from build123d import *

# Parameters (mm, degrees)
SKETCH1_R           = 3.2512
SKETCH1_R_2         = 1.27
BOSS_EXTRUDE1_DEPTH = 0.800000051


with BuildPart() as part:
    # Sketch1 → Boss-Extrude1 (new body)
    with BuildSketch(Plane.XY):
        with BuildLine():
            ThreePointArc((21.253467287, -26.289), (46.841342124, -13.11656107), (18.612068966, -7.516505446))
            ThreePointArc((18.612068966, -7.516505446), (15.875, -9.08244408), (13.137931034, -7.516505446))
            ThreePointArc((13.137931034, -7.516505446), (-15.091342124, -13.11656107), (10.496532713, -26.289))
            Line((10.496532713, -26.289), (21.253467287, -26.289))
        make_face()
        with Locations(Location((31.75, -15.24, 0), (0, 0, 180))):
            Circle(SKETCH1_R, mode=Mode.SUBTRACT)
        with Locations(Location((0, -15.24, 0), (0, 0, 180))):
            Circle(SKETCH1_R, mode=Mode.SUBTRACT)
        with Locations(Location((-11.733270063, -10.379920409, 0), (0, 0, 180))):
            Circle(SKETCH1_R_2, mode=Mode.SUBTRACT)
        with Locations(Location((11.733270063, -10.379920409, 0), (0, 0, 180))):
            Circle(SKETCH1_R_2, mode=Mode.SUBTRACT)
        with Locations(Location((-4.860079591, -3.506729937, 0), (0, 0, 180))):
            Circle(SKETCH1_R_2, mode=Mode.SUBTRACT)
        with Locations(Location((4.860079591, -3.506729937, 0), (0, 0, 180))):
            Circle(SKETCH1_R_2, mode=Mode.SUBTRACT)
        with Locations(Location((20.016729937, -10.379920409, 0), (0, 0, 180))):
            Circle(SKETCH1_R_2, mode=Mode.SUBTRACT)
        with Locations(Location((43.483270063, -10.379920409, 0), (0, 0, 180))):
            Circle(SKETCH1_R_2, mode=Mode.SUBTRACT)
        with Locations(Location((26.889920409, -3.506729937, 0), (0, 0, 180))):
            Circle(SKETCH1_R_2, mode=Mode.SUBTRACT)
        with Locations(Location((36.610079591, -3.506729937, 0), (0, 0, 180))):
            Circle(SKETCH1_R_2, mode=Mode.SUBTRACT)
        with Locations(Location((36.610079591, -26.973270063, 0), (0, 0, 180))):
            Circle(SKETCH1_R_2, mode=Mode.SUBTRACT)
        with Locations(Location((20.016729937, -20.100079591, 0), (0, 0, 180))):
            Circle(SKETCH1_R_2, mode=Mode.SUBTRACT)
        with Locations(Location((43.483270063, -20.100079591, 0), (0, 0, 180))):
            Circle(SKETCH1_R_2, mode=Mode.SUBTRACT)
        with Locations(Location((-4.860079591, -26.973270063, 0), (0, 0, 180))):
            Circle(SKETCH1_R_2, mode=Mode.SUBTRACT)
        with Locations(Location((4.860079591, -26.973270063, 0), (0, 0, 180))):
            Circle(SKETCH1_R_2, mode=Mode.SUBTRACT)
        with Locations(Location((-11.733270063, -20.100079591, 0), (0, 0, 180))):
            Circle(SKETCH1_R_2, mode=Mode.SUBTRACT)
        with Locations(Location((11.733270063, -20.100079591, 0), (0, 0, 180))):
            Circle(SKETCH1_R_2, mode=Mode.SUBTRACT)
        with Locations(Location((26.889920409, -26.973270063, 0), (0, 0, 180))):
            Circle(SKETCH1_R_2, mode=Mode.SUBTRACT)
    extrude(amount=BOSS_EXTRUDE1_DEPTH)


solid = part.part
Model file for the job. Use its own axes, mm. Give positions to 0.01 mm unless a question says otherwise; leave off trailing zeros. Order: outer loops, then holes, each group sorted by start corner. A loop starts at its lowest first (then second) coordinate and runs counter-clockwise, first axis right, second up. Notation, with made-up numbers: (60.25, 52.5) - (113.25, 52.5) arc R9 cw to (113.25, 59.5) - close; hole circle Ø3 at (64, 72). An arc over 180 degrees is marked (long way). Return JSON: item names as keys, results as strings.
1) Probe line 1 (Y direction, x = 37, z = 0.65); line 2 (X direction, y = -15.24, z = 0.45); line 3 (X direction, y = -4, z = 0.75). List the from-to ranges inside material, lowest first. Write a range as from..to.
Geometry says:
{"line 1": "-29.55..-28.18, -25.76..-4.72, -2.3..-0.93", "line 2": "-15.24..-3.25, 3.25..28.5, 35..46.99", "line 3": "-10.29..-6.03, -3.69..3.69, 6.03..10.29, 21.46..25.72, 28.06..35.44, 37.78..42.04"}
2) Cut at A-A, the plane y = -15.24. Give the cut face in (x, z).
Geometry says:
{"outline": "(-15.24, 0) - (-3.25, 0) - (-3.25, 0.8) - (-15.24, 0.8) - close; (3.25, 0) - (28.5, 0) - (28.5, 0.8) - (3.25, 0.8) - close; (35, 0) - (46.99, 0) - (46.99, 0.8) - (35, 0.8) - close"}
3) Pull direction Y, two halves, no side cores. Call faces 1 (the cylindrical face through (2.396, -17.437, 0.394)), 2 (the cylindrical face through (15.921, -9.082, 0.394)), 3 (the cylindrical face through (46.9, -13.6, 0.4)): pulls with the +Y half, pulls with the -Y half, needs draft (parallel to the pull), parting line crosses it, or undercut.
Geometry says:
{"face 1": "undercut", "face 2": "pulls with the +Y half", "face 3": "parting line crosses it"}
4) Cut at D-D, the plane y = -19.5. Give the cut face in (x, z), plus the area to 3 significant figures.
Geometry says:
{"outline": "(-14.63, 0) - (-12.85, 0) - (-12.85, 0.8) - (-14.63, 0.8) - close; (-10.61, 0) - (10.61, 0) - (10.61, 0.8) - (-10.61, 0.8) - close; (12.85, 0) - (18.9, 0) - (18.9, 0.8) - (12.85, 0.8) - close; (21.14, 0) - (42.36, 0) - (42.36, 0.8) - (21.14, 0.8) - close; (44.6, 0) - (46.38, 0) - (46.38, 0.8) - (44.6, 0.8) - close", "area": "41.6 mm²"}
5) Cut at C-C, the plane z = 0.5. Count the separate pieces of the cut face and the enclosed holes in it, plus the area to 3 significant figures.
Geometry says:
{"separate pieces": "1", "enclosed holes": "18", "area": "1,370 mm²"}
6) Cut at B-B, the plane x = 31.75. Give the cut face in (y, z), plus the area to 3 significant figures.
Geometry says:
{"outline": "(-30.48, 0) - (-18.49, 0) - (-18.49, 0.8) - (-30.48, 0.8) - close; (-11.99, 0) - (0, 0) - (0, 0.8) - (-11.99, 0.8) - close", "area": "19.2 mm²"}
